```python
from build123d import *

# Parameters (mm, degrees)
ESQUISSE1_R             = 12.5
BOSS_EXTRU_1_DEPTH      = 80
BOSS_EXTRU_2_DEPTH      = 90
BOSS_EXTRU_2_DEPTH_BACK = 20
ESQUISSE2_R             = 2.5
CONG_1_R                = 2
CONG_2_R                = 2
ENL_V_START             = -5
ESQUISSE3_R             = 0.5
ENL_V_MAT_EXTRU_1_DEPTH = 90
ENL_V_MAT_EXTRU_3_DEPTH = 1


with BuildPart() as part:
    # Esquisse1 → Boss.-Extru.1 (new body)
    with BuildSketch(Plane.XY):
        Circle(ESQUISSE1_R)
    extrude(amount=BOSS_EXTRU_1_DEPTH)

    # Esquisse2 → Boss.-Extru.2 (add, two sides: drawn at the far end of the back side and taken through both)
    with BuildSketch(Plane.XY.offset(-BOSS_EXTRU_2_DEPTH_BACK)):
        with Locations(Location((0, 0, 0), (0, 0, 180))):
            Circle(ESQUISSE2_R)
    extrude(amount=BOSS_EXTRU_2_DEPTH + BOSS_EXTRU_2_DEPTH_BACK)

    # Congé1
    cong_1_edges = [part.edges().sort_by_distance(p)[0] for p in [
        (2.5, 0, 80),
    ]]
    fillet(cong_1_edges, radius=CONG_1_R)

    # Congé2
    cong_2_edges = [part.edges().sort_by_distance(p)[0] for p in [
        (2.5, 0, 0),
    ]]
    fillet(cong_2_edges, radius=CONG_2_R)

    # Esquisse3 → Enlèv. mat.-Extru.1 (cut)
    with BuildSketch(Plane.XY.offset(90).offset(ENL_V_START)):
        Circle(ESQUISSE3_R)
    extrude(amount=-ENL_V_MAT_EXTRU_1_DEPTH, mode=Mode.SUBTRACT)

    # Esquisse5 → Enlèv. mat.-Extru.3 (cut)
    with BuildSketch(Plane.XY.offset(90)):
        with BuildLine():
            Line((-2.449489743, -0.5), (2.449489743, -0.5))
            ThreePointArc((2.449489743, -0.5), (2.5, 0), (2.449489743, 0.5))
            Line((2.449489743, 0.5), (-2.449489743, 0.5))
            ThreePointArc((-2.449489743, 0.5), (-2.5, 0), (-2.449489743, -0.5))
        make_face()
    extrude(amount=-ENL_V_MAT_EXTRU_3_DEPTH, mode=Mode.SUBTRACT)


solid = part.part
```
The model under review builds one solid part; all positions refer to its coordinate system, in mm. A direction names the side the tool comes from. Round coordinates to 2 decimals unless told otherwise and drop trailing zeros. Loops run counter-clockwise (first coordinate to the right, second up) from the corner with the lowest first, then second, coordinate; pieces in that order, holes last. Notation, with made-up numbers: M 21.5,49 L 53.5,49 A13 ccw 53.5,64 Z; hole C 23,21 d9. An arc over 180 degrees is marked long. Answer as a JSON object with one key per item and string values.
(1) Take a section at B-B on z = -8.5. Give the boundary of the cut face in (x, y), and give its area (3 significant figures).
Resolved:
{"outline": "C 0,0 d5", "area": "19.6 mm²"}
(2) To check wall thickness, follow line 1 along Y through (x, z) = (0, 31); line 2 along Z through (x, y) = (-6.25, -6); line 3 along X through (y, z) = (0.25, 40.5). State the ranges of each line that lie inside material, in increasing order.
Resolved:
{"line 1": "-12.5 to -0.5, 0.5 to 12.5", "line 2": "0 to 80", "line 3": "-12.5 to -0.43, 0.43 to 12.5"}
(3) Take a section at C-C on x = 9. Give the boundary of the cut face in (y, z), and give its area (3 significant figures).
Resolved:
{"outline": "M -8.67,0 L 8.67,0 L 8.67,80 L -8.67,80 Z", "area": "1,390 mm²"}
(4) Take a section at D-D on y = 10.25. Give the boundary of the cut face in (x, z), and give its area (3 significant figures).
Resolved:
{"outline": "M -7.15,0 L 7.15,0 L 7.15,80 L -7.15,80 Z", "area": "1,140 mm²"}
(5) Take a section at A-A on z = 3. Give the boundary of the cut face in (x, y).
Resolved:
{"outline": "C 0,0 d25; hole C 0,0 d1"}
(6) Tool access review of faces 1 (the flat face through (0, -5, 0)), 2 (the flat face through (0, -5, 80)), 3 (the flat face through (0, 0, -20)): name each direction out of +Z, -Z, +X, -X, +Y, -Y from which nothing blocks a thin tool from reaching the whole face with its end or side.
Resolved:
{"face 1": "-Z", "face 2": "+Z", "face 3": "-Z, +X, -X, +Y, -Y"}
(7) Clearance check with flat-ended pins moving along their axes: P1, Ø1, axis at x = -2, z = 21.5, coming from the +Y side; P2, Ø2, axis at x = -5, y = 7, coming from the -Z side; P3, Ø3, axis at x = -2, z = 66, coming from the -Y side; P4, Ø1, axis at y = -10, z = -1.5, coming from the +X side. State where each tip first meets the part, or that it passes through.
Resolved:
{"P1": "y = 12.41", "P2": "z = 0", "P3": "y = -12.49", "P4": "through"}
